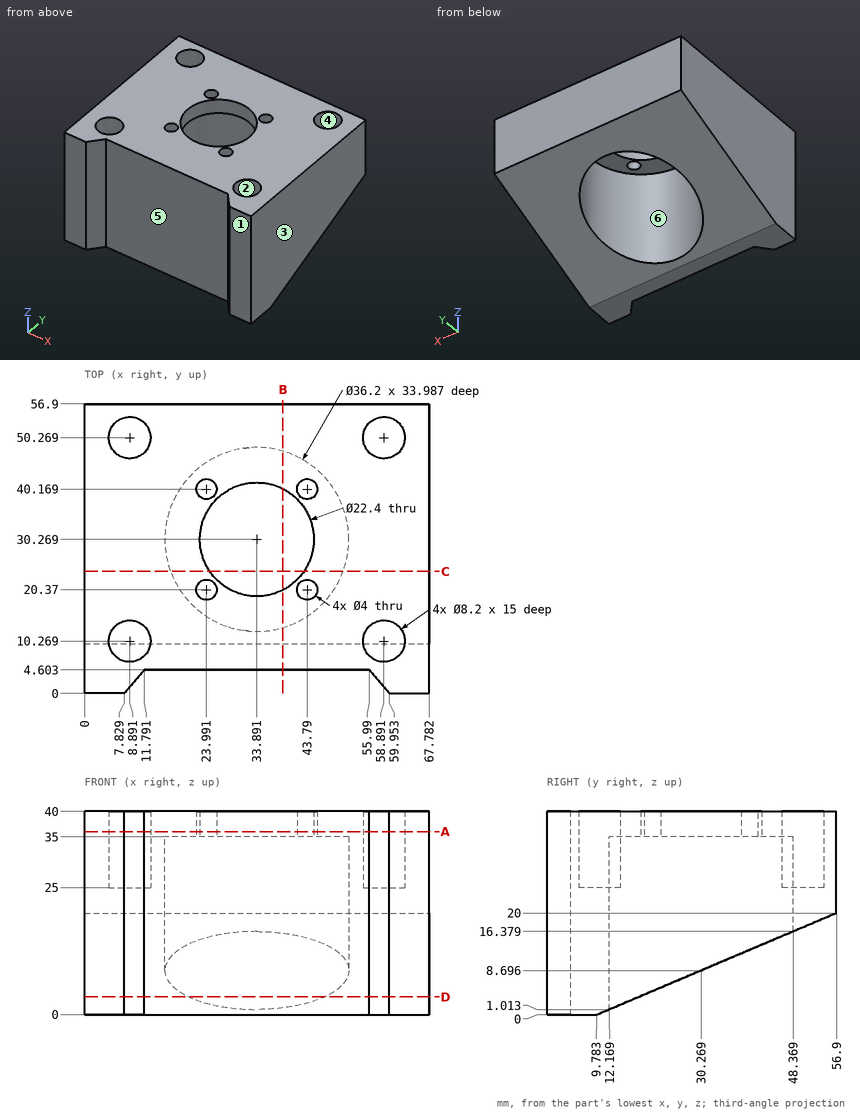
Geometry check sheet. Reference: drawing and pictorial views, mm from the part's lowest x, y, z. A direction names the side the tool comes from. Coordinates: 2 decimals unless noted, no trailing zeros. Order: outer loops, then holes, each group sorted by start corner. A loop starts at its lowest first (then second) coordinate and runs counter-clockwise, first axis right, second up. Notation, with made-up numbers: M 68.5,57.5 L 97.5,57.5 A20 cw 97.5,91.5 Z; hole C 8.25,72 d7. An arc over 180 degrees is marked long. Return JSON: item names as keys, results as strings.
1) Release check for a two-part mould opening along X. For the marked faces 1, 2 and 3 record: +X half, -X half, draft (parallel to the pull), parting line (faces both ways), or undercut.
Answer list:
{"face 1": "draft", "face 2": "undercut", "face 3": "+X half"}
2) Cross-section at D-D, the plane z = 3.5. Record the boundary of the cut face in (x, y).
Answer list:
{"outline": "M 0,0 L 7.83,0 L 11.79,4.6 L 55.99,4.6 L 59.95,0 L 67.78,0 L 67.78,18.03 L 47.22,18.03 A18.1 cw 20.56,18.03 L 0,18.03 Z"}
3) Access from +Z, -Z, +X, -X, +Y, -Y to the whole of each face (thin tool, end or side, straight path). Record for the marked faces 4, 5 and 6.
Answer list:
{"face 4": "+Z", "face 5": "+Z, -Z, -Y", "face 6": "-Z"}
4) Cross-section at B-B, the plane x = 39. Record the boundary of the cut face in (y, z) (1 decimal).
Answer list:
{"outline": "M 4.6,0 L 9.8,0 L 12.9,1.3 L 12.9,35 L 20.3,35 L 20.3,40 L 4.6,40 Z; M 40.2,35 L 47.6,35 L 47.6,16.1 L 56.9,20 L 56.9,40 L 40.2,40 Z"}
5) Thickness scan on L1, parallel to Y at x = 15, z = 26; L2, parallel to Y at x = 10.5, z = 33.5 (1 decimal); L3, parallel to Z at x = 36.5, y = 14.5. Record the ranges inside material, lowest first. Write a range as [from, to].
Answer list:
{"L1": "[4.6, 56.9]", "L2": "[3.1, 6.5], [14, 46.5], [54, 56.9]", "L3": "[35, 40]"}
6) Cross-section at A-A, the plane z = 36. Count the separate pieces of the cut face and the enclosed holes in it, and give its area (3 significant figures).
Answer list:
{"separate pieces": "1", "enclosed holes": "9", "area": "2,980 mm2"}
7) Cross-section at C-C, the plane y = 24. Record the boundary of the cut face in (x, z) (1 decimal), and give its area (3 significant figures).
Answer list:
{"outline": "M 0,6 L 16.9,6 L 16.9,35 L 24.6,35 L 24.6,40 L 0,40 Z; M 43.2,35 L 50.9,35 L 50.9,6 L 67.8,6 L 67.8,40 L 43.2,40 Z", "area": "1,230 mm2"}
8) Gauge pin test, flat ends, axial feed: pin 1 (10.5 mm diameter, centred on x = 8.89, y = 50.27, fed in from -Z); pin 2 (9.5 mm diameter, centred on x = 58.89, y = 50.27, fed in from -Z); pin 3 (5 mm diameter, centred on x = 23.99, y = 20.37, fed in from -Z). Record the tip position at first contact, or that the pin passes through.
Answer list:
{"pin 1": "z = 14.96", "pin 2": "z = 15.17", "pin 3": "z = 35"}
